Source: CAD feature listing. Evaluate the final solid. Frame: model axes, mm. Face numbers are marked on the shaded views. Coordinates: 2 decimals unless noted, no trailing zeros. Order: outer loops, then holes, each group sorted by start corner. A loop starts at its lowest first (then second) coordinate and runs counter-clockwise, first axis right, second up. Notation, with made-up numbers: (24.25, -29.5) - (67.25, -29.5) arc R29 ccw to (67.25, -3.5) - close; hole circle Ø5 at (46, -12). An arc over 180 degrees is marked (long way). One line per question, with ' | ' between items.
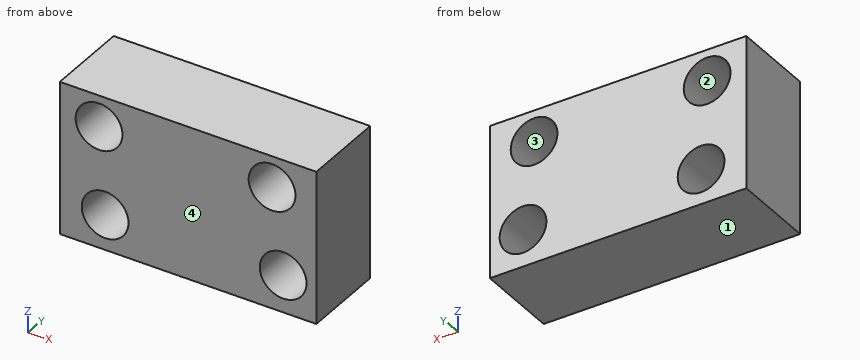
from build123d import *

# Parameters (mm, degrees)
F0_W     = 77.724002
F0_H     = 46.329598
F0_R     = 7.0866
F0_R_2   = 7.089467
F1_DEPTH = 25.4


with BuildPart() as f1:
    # F0 (on Front) → F1 (new body)
    with BuildSketch(Plane.XZ):
        Rectangle(F0_W, F0_H)
        with Locations((-25.146, -12.496799)):
            Circle(F0_R, mode=Mode.SUBTRACT)
        with Locations((28.803604, -11.8872)):
            Circle(F0_R, mode=Mode.SUBTRACT)
        with Locations((-26.974799, 13.716)):
            Circle(F0_R_2, mode=Mode.SUBTRACT)
        with Locations((25.450798, 13.716)):
            Circle(F0_R, mode=Mode.SUBTRACT)
    extrude(amount=F1_DEPTH)


solid = f1.part
(1) Cut plane A-A (z = -14). Return the cut outline in (x, y), and give its area (3 significant figures).
Taken from the geometry:
outline: (-38.86, -25.4) - (-32.07, -25.4) - (-32.07, 0) - (-38.86, 0) - close; (-18.22, -25.4) - (22.04, -25.4) - (22.04, 0) - (-18.22, 0) - close; (35.57, -25.4) - (38.86, -25.4) - (38.86, 0) - (35.57, 0) - close | area: 1,280 mm²
(2) Pull-direction query (Z, two-part tool) for the marked faces 1, 2, 3 and 4; classes: pulls with the +Z half, pulls with the -Z half, needs draft (parallel to the pull), parting line crosses it, or undercut.
Taken from the geometry:
face 1: pulls with the -Z half | face 2: undercut | face 3: undercut | face 4: needs draft
(3) Material intervals for L1, parallel to Z at x = 32, y = -20.5; L2, parallel to X at y = -21, z = -14.5; L3, parallel to X at y = -14, z = 8.5, sorted ascending. Write a range as from..to.
Taken from the geometry:
L1: z = -23.16..-18.21, -5.56..11.01, 16.42..23.16 | L2: x = -38.86..-31.94, -18.35..22.22, 35.39..38.86 | L3: x = -38.86..-31.78, -22.17..20.65, 30.25..38.86
(4) Cut plane B-B (x = -19). Return the cut outline in (y, z).
Taken from the geometry:
outline: (-25.4, -23.16) - (0, -23.16) - (0, -16.02) - (-25.4, -16.02) - close; (-25.4, -8.97) - (0, -8.97) - (0, 23.16) - (-25.4, 23.16) - close
(5) Pin query (flat end, axial travel): P1, Ø11.5, axis at x = -25.15, z = -12.5, coming from the +Y side. Return the tip coordinate at first contact, or that it passes through.
Taken from the geometry:
P1: passes through
(6) Cut plane C-C (y = -17). Return the cut outline in (x, z).
Taken from the geometry:
outline: (-38.86, -23.16) - (38.86, -23.16) - (38.86, 23.16) - (-38.86, 23.16) - close; hole circle Ø14.18 at (-26.97, 13.72); hole circle Ø14.17 at (-25.15, -12.5); hole circle Ø14.17 at (25.45, 13.72); hole circle Ø14.17 at (28.8, -11.89)
(7) Cut plane D-D (x = 24). Return the cut outline in (y, z), and give its area (3 significant figures).
Taken from the geometry:
outline: (-25.4, -23.16) - (0, -23.16) - (0, -17.1) - (-25.4, -17.1) - close; (-25.4, -6.68) - (0, -6.68) - (0, 6.78) - (-25.4, 6.78) - close; (-25.4, 20.65) - (0, 20.65) - (0, 23.16) - (-25.4, 23.16) - close | area: 560 mm²
